Could you check a few things on this model? Use its own coordinates, in mm. Round coordinates to 2 decimals unless told otherwise and drop trailing zeros. Write each loop counter-clockwise with the first axis right and the second up, starting at its lowest first coordinate (ties: lowest second). Pieces come first, ordered by that corner, then holes. Notation, with made-up numbers: (-24.75, 59) -> (5.25, 59) arc R30 cw to (5.25, 83) -> close; hole circle Ø8 at (-32, -8.5). An arc over 180 degrees is marked (long way). Answer in a Markdown table with one row per item.
from build123d import *

# Parameters (mm, degrees)
SKETCH1_W           = 5.08
SKETCH1_H           = 6.35
SKETCH1_W_2         = 118.745
SKETCH1_H_2         = 44.45
SKETCH1_R           = 10.668
BOSS_EXTRUDE1_DEPTH = 5.08


with BuildPart() as part:
    # Sketch1 → Boss-Extrude1 (new body)
    with BuildSketch(Plane(origin=(0, 0, 0), x_dir=(1, 0, 0), z_dir=(0, 1, 0))):
        with Locations((-61.9125, -19.05)):
            Rectangle(SKETCH1_W, SKETCH1_H)
        with Locations((-61.9125, 19.05)):
            Rectangle(SKETCH1_W, SKETCH1_H)
        Rectangle(SKETCH1_W_2, SKETCH1_H_2)
        with Locations((-11.7475, 0)):
            Circle(SKETCH1_R, mode=Mode.SUBTRACT)
        with Locations((61.9125, 19.05)):
            Rectangle(SKETCH1_W, SKETCH1_H)
        with Locations((61.9125, -19.05)):
            Rectangle(SKETCH1_W, SKETCH1_H)
    extrude(amount=BOSS_EXTRUDE1_DEPTH)


solid = part.part
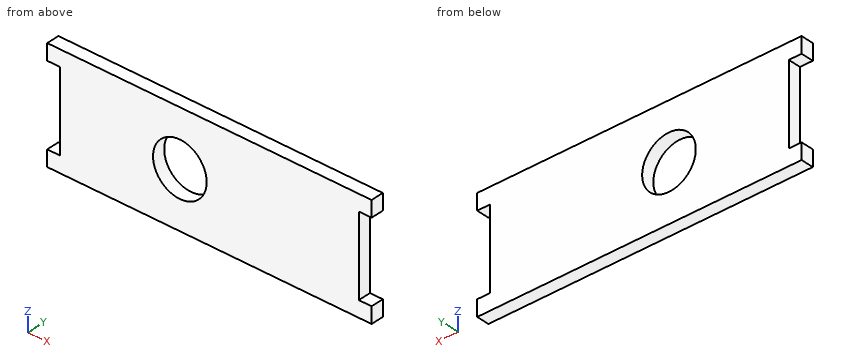
1) For pin 1 (2.5 mm diameter, centred on y = 2, z = -7, fed in from +X); pin 2 (3 mm diameter, centred on y = 4, z = 11.5, fed in from -X), each with a flat end and sliding along its axis, tell me the tip position at first contact or that it passes through.
Findings:
| item | result |
|---|---|
| pin 1 | stops at x = 59.37 |
| pin 2 | stops at x = -59.37 |
2) Please list where these lines run through material, in increasing order: line 1 (X direction, y = 2, z = 0); line 2 (X direction, y = 3.65, z = 15.5); line 3 (Z direction, x = -6.5, y = 3.9) (3 decimals).
Findings:
| item | result |
|---|---|
| line 1 | x = -59.37 to -22.42, -1.08 to 59.37 |
| line 2 | x = -59.37 to 59.37 |
| line 3 | z = -22.225 to -9.288, 9.288 to 22.225 |
3) Imagine slicing it at A-A, the plane y = 2.15. Please give me the cut outline in (x, z) (1 decimal).
Findings:
| item | result |
|---|---|
| outline | (-64.5, -22.2) -> (64.5, -22.2) -> (64.5, -15.9) -> (59.4, -15.9) -> (59.4, 15.9) -> (64.5, 15.9) -> (64.5, 22.2) -> (-64.5, 22.2) -> (-64.5, 15.9) -> (-59.4, 15.9) -> (-59.4, -15.9) -> (-64.5, -15.9) -> close; hole circle Ø21.3 at (-11.7, 0) |
4) Imagine slicing it at B-B, the plane z = 0. Please give me the cut outline in (x, y), plus the area to 3 significant figures.
Findings:
| item | result |
|---|---|
| outline | (-59.37, 0) -> (-22.42, 0) -> (-22.42, 5.08) -> (-59.37, 5.08) -> close; (-1.08, 0) -> (59.37, 0) -> (59.37, 5.08) -> (-1.08, 5.08) -> close |
| area | 495 mm^2 |
5) Imagine slicing it at C-C, the plane z = -8.5. Please give me the cut outline in (x, y), plus the area to 3 significant figures.
Findings:
| item | result |
|---|---|
| outline | (-59.37, 0) -> (-18.19, 0) -> (-18.19, 5.08) -> (-59.37, 5.08) -> close; (-5.3, 0) -> (59.37, 0) -> (59.37, 5.08) -> (-5.3, 5.08) -> close |
| area | 538 mm^2 |
